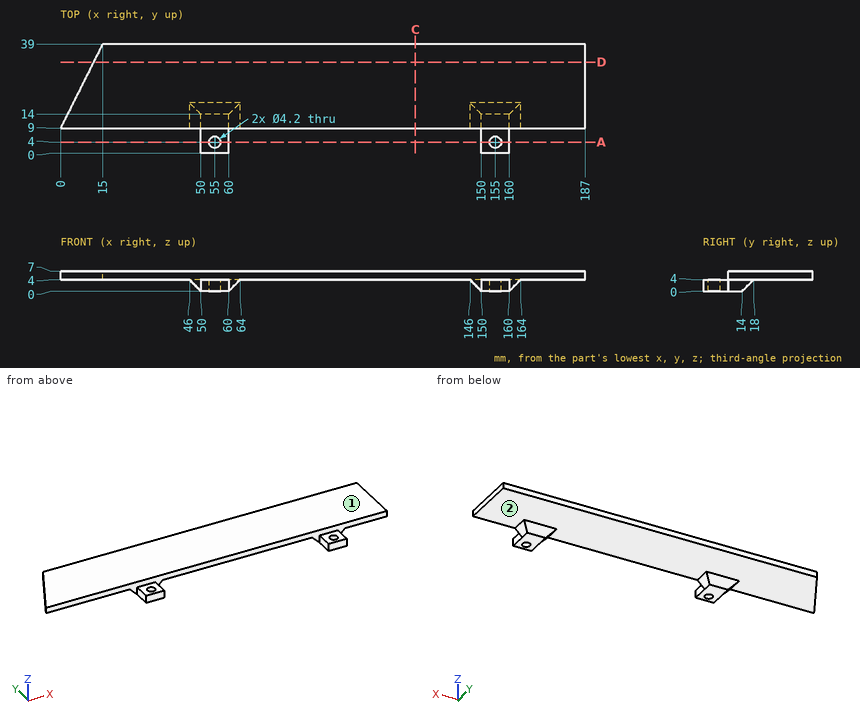
Input: dimensioned drawing with shaded views. Units: mm. Origin: part minimum x, y, z. A direction names the side the tool comes from. Round coordinates to 2 decimals unless told otherwise and drop trailing zeros. Loops run counter-clockwise (first coordinate to the right, second up) from the corner with the lowest first, then second, coordinate; pieces in that order, holes last. Notation, with made-up numbers: (23.5, 56) -> (79.5, 56) arc R13 ccw to (79.5, 72) -> close; hole circle Ø3 at (-14.75, 84.25). An arc over 180 degrees is marked (long way). Answer as a JSON object with one key per item and string values. Group by question number.
1) Pin query (flat end, axial travel): pin 1 (9 mm diameter, centred on x = 52.5, y = 24.5, fed in from -Z); pin 2 (5 mm diameter, centred on x = 66, y = 4.5, fed in from +Z); pin 3 (2 mm diameter, centred on y = 14.5, z = 4.5, fed in from -X); pin 4 (4.5 mm diameter, centred on x = 152.5, y = 6, fed in from +Z). Return the tip coordinate at first contact, or that it passes through.
2) Section query D-D on y = 32.5. Output: boundary loops of the cut face in (x, z), plus the area to 3 significant figures.
3) Section query A-A on y = 4. Output: boundary loops of the cut face in (x, z), plus the area to 3 significant figures.
4) Section query C-C on x = 126.5. Output: boundary loops of the cut face in (y, z), plus the area to 3 significant figures.
5) Ray query, L1, parallel to X at y = 7, z = 1.25; L2, parallel to Z at x = 93, y = 13.5; L3, parallel to Y at x = 155, z = 2.75. Return the intervals inside material, ascending.
6) Reachability of the marked faces 1 and 2 from +Z, -Z, +X, -X, +Y, -Y: full face, straight path, thin tool, end or side. Return the list, or none.
Reply:
{
 "1": {"pin 1": "stops at z = 4", "pin 2": "passes through", "pin 3": "stops at x = 2.25", "pin 4": "stops at z = 4"},
 "2": {"outline": "(11.75, 4) -> (187, 4) -> (187, 7) -> (11.75, 7) -> close", "area": "526 mm2"},
 "3": {"outline": "(50, 0) -> (52.9, 0) -> (52.9, 4) -> (50, 4) -> close; (57.1, 0) -> (60, 0) -> (60, 4) -> (57.1, 4) -> close; (150, 0) -> (152.9, 0) -> (152.9, 4) -> (150, 4) -> close; (157.1, 0) -> (160, 0) -> (160, 4) -> (157.1, 4) -> close", "area": "46.4 mm2"},
 "4": {"outline": "(9, 4) -> (39, 4) -> (39, 7) -> (9, 7) -> close", "area": "90.0 mm2"},
 "5": {"L1": "x = 50 to 60, 150 to 160", "L2": "z = 4 to 7", "L3": "y = 0 to 1.9, 6.1 to 16.75"},
 "6": {"face 1": "+Z, +X, -X, +Y, -Y", "face 2": "-Z, +Y"}
}
